from build123d import *

# Parameters (mm, degrees)
EXTRUDE_1_DEPTH     = 10
SKETCH_1_15_R       = 1.62
CUT_EXTRUDE_2_DEPTH = 10
SKETCH_1_16_R       = 9.8
CUT_EXTRUDE_3_DEPTH = 2.2


with BuildPart() as part:
    # Sketch 1 → Extrude 1 (new body)
    with BuildSketch(Plane.XY):
        with BuildLine():
            Line((-150, -1.5), (-150, -8.5))
            ThreePointArc((-150, -8.5), (-149.560660172, -9.560660172), (-148.5, -10))
            Line((-148.5, -10), (1.474010293, -10))
            ThreePointArc((1.474010293, -10), (7.366779588, -19.192759664), (18.180300258, -17.676405182))
            Line((18.180300258, -17.676405182), (26.670550932, -11.495316766))
            ThreePointArc((26.670550932, -11.495316766), (29.697133836, -7.946431766), (30.784873277, -3.410837899))
            Line((30.784873277, -3.410837899), (30.784873277, -1.622776602))
            ThreePointArc((30.784873277, -1.622776602), (30.9139987, -0.020954172), (31.298040296, 1.539501058))
            Line((31.298040296, 1.539501058), (59.329162551, 85.632867822))
            ThreePointArc((59.329162551, 85.632867822), (50.093700568, 104.103791788), (31.622776602, 94.868329805))
            Line((31.622776602, 94.868329805), (0, 0))
            Line((0, 0), (-148.5, 0))
            ThreePointArc((-148.5, 0), (-149.560660172, -0.439339828), (-150, -1.5))
        make_face()
    extrude(amount=EXTRUDE_1_DEPTH)

    # Sketch 1_15 → Cut-Extrude 2 (cut)
    with BuildSketch(Plane.XY):
        with Locations((44.787529943, 88.101420291)):
            Circle(SKETCH_1_15_R)
        with Locations((51.946529943, 88.101420291)):
            Circle(SKETCH_1_15_R)
        with Locations((44.787529943, 95.260420291)):
            Circle(SKETCH_1_15_R)
        with Locations(Location((44.787529943, 80.942420291, 0), (0, 0, 180))):
            Circle(SKETCH_1_15_R)
        with Locations(Location((37.628529943, 88.101420291, 0), (0, 0, 180))):
            Circle(SKETCH_1_15_R)
    extrude(amount=CUT_EXTRUDE_2_DEPTH, mode=Mode.SUBTRACT)

    # Sketch 1_16 → Cut-Extrude 3 (cut)
    with BuildSketch(Plane.XY):
        with Locations((44.787529943, 88.101420291)):
            Circle(SKETCH_1_16_R)
    extrude(amount=CUT_EXTRUDE_3_DEPTH, mode=Mode.SUBTRACT)


solid = part.part
Verification items for the finished model (mm, model axes). A direction names the side the tool comes from. Round coordinates to 2 decimals unless told otherwise and drop trailing zeros. Loops run counter-clockwise (first coordinate to the right, second up) from the corner with the lowest first, then second, coordinate; pieces in that order, holes last. Notation, with made-up numbers: (-3.5, 6) - (20.5, 6) arc R6 ccw to (20.5, 10) - close; hole circle Ø4 at (14, -28.5). An arc over 180 degrees is marked (long way). Use a Markdown table: item, result. Add a question column.
1. Gauge pin test, flat ends, axial feed: pin 1 (3 mm diameter, centred on x = -57, z = 5.5, fed in from -Y); pin 2 (5 mm diameter, centred on x = 44.79, y = 80.94, fed in from +Z); pin 3 (5 mm diameter, centred on x = 44.79, y = 88.1, fed in from -Z); pin 4 (1.5 mm diameter, centred on x = -89.5, z = 6.5, fed in from +Y). Record the tip position at first contact, or that the pin passes through.
2. Section check A-A, the plane x = -73. Record the boundary of the cut face in (y, z), plus the area to 3 significant figures.
3. Section check B-B, the plane z = 7.5. Record the boundary of the cut face in (x, y), plus the area to 3 significant figures.
4. Section check C-C, the plane y = 14. Record the boundary of the cut face in (x, z), plus the area to 3 significant figures.
5. Thickness scan on probe 1 along X at (y, z) = (-11.5, 4.25); probe 2 along Y at (x, z) = (-30.5, 7.5); probe 3 along X at (y, z) = (-4, 1.75). Record the ranges inside material, lowest first. Write a range as [from, to].
6. Access from +Z, -Z, +X, -X, +Y, -Y to the whole of each face (thin tool, end or side, straight path). Record for faces 1 (the face through (-73, 0, 5)), 2 (the face through (9, 20, 10)), 3 (the face through (-75, -10, 5)).
7. Release check for a two-part mould opening along X. For faces 4 (the face through (50.4, 104, 4.9)), 5 (the face through (45, 86, 2.2)), 6 (the face through (42.663, 78.534, 1.085)), 7 (the face through (9, 24, 0)) record: released by +X, released by -X, zero draft, split by the parting line, or undercut.
Checks:
| question | item | result |
|---|---|---|
| 1 | pin 1 | stops at y = -10 |
| 1 | pin 2 | stops at z = 10 |
| 1 | pin 3 | stops at z = 2.2 |
| 1 | pin 4 | stops at y = 0 |
| 2 | outline | (-10, 0) - (0, 0) - (0, 10) - (-10, 10) - close |
| 2 | area | 100 mm^2 |
| 3 | outline | (-150, -8.5) arc R1.5 ccw to (-148.5, -10) - (1.47, -10) arc R10.12 ccw to (18.18, -17.68) - (26.67, -11.5) arc R10 ccw to (30.78, -3.41) - (30.78, -1.62) arc R10 cw to (31.3, 1.54) - (59.33, 85.63) arc R14.6 ccw to (31.62, 94.87) - (0, 0) - (-148.5, 0) arc R1.5 ccw to (-150, -1.5) - close; hole circle Ø3.24 at (37.63, 88.1); hole circle Ø3.24 at (44.79, 80.94); hole circle Ø3.24 at (44.79, 88.1); hole circle Ø3.24 at (44.79, 95.26); hole circle Ø3.24 at (51.95, 88.1) |
| 3 | area | 5,060 mm^2 |
| 4 | outline | (4.67, 0) - (35.45, 0) - (35.45, 10) - (4.67, 10) - close |
| 4 | area | 308 mm^2 |
| 5 | probe 1 | x = [1.59, 26.66] |
| 5 | probe 2 | y = [-10, 0] |
| 5 | probe 3 | x = [-150, 30.77] |
| 6 | face 1 | +Z, -Z, -X, +Y |
| 6 | face 2 | +Z, +X, -X, +Y, -Y |
| 6 | face 3 | +Z, -Z, -X, -Y |
| 7 | face 4 | split by the parting line |
| 7 | face 5 | undercut |
| 7 | face 6 | undercut |
| 7 | face 7 | zero draft |
